Job drawing, mm, ordinate dimensions from the low corner. One solid piece. A direction names the side the tool comes from. Coordinates: 2 decimals unless noted, no trailing zeros. Order: outer loops, then holes, each group sorted by start corner. A loop starts at its lowest first (then second) coordinate and runs counter-clockwise, first axis right, second up. Notation, with made-up numbers: (78, -21) -> (99, -21) arc R26 cw to (99, 2) -> close; hole circle Ø6 at (3.5, 48.5). An arc over 180 degrees is marked (long way). Use CSV: the item, a comma, the result in double quotes. Start each with the question number.
(1) Cut at C-C on y = 13. Write the cut outline in (x, z), plus the area to 3 significant figures.
(2) Cut at D-D on y = 5.5. Write the cut outline in (x, z) (3 decimals), plus the area to 3 significant figures.
(3) Cut at B-B on z = 17.5. Write the cut outline in (x, y) (3 decimals).
(4) Tool access for the marked faces 4 and 5: list every direction of +Z, -Z, +X, -X, +Y, -Y with a clear straight run to the whole face (end or side of a thin tool).
(5) Cut at A-A on x = 17.5. Write the cut outline in (y, z) (3 decimals).
(6) Pin check, flat tips, straight feed: pin 1 Ø8 at (x, z) = (17.5, 17.5) entering from -Y; pin 2 Ø3 at (x, y) = (11.5, 4.5) entering from +Z; pin 3 Ø8 at (x, y) = (24.5, 12) entering from +Z. Stop position of each tip, or through.
(7) Probe L1, parallel to Y at x = 26, z = 13.5; L2, parallel to Z at x = 17.5, y = 5.25 (3 decimals); L3, parallel to Z at x = 17.5, y = 16.5 (3 decimals). List the from-to ranges inside material, lowest first.
(8) Pull direction X, two halves, no side cores. Call the marked faces 1, 2 and 3: pulls with the +X half, pulls with the -X half, needs draft (parallel to the pull), parting line crosses it, or undercut.
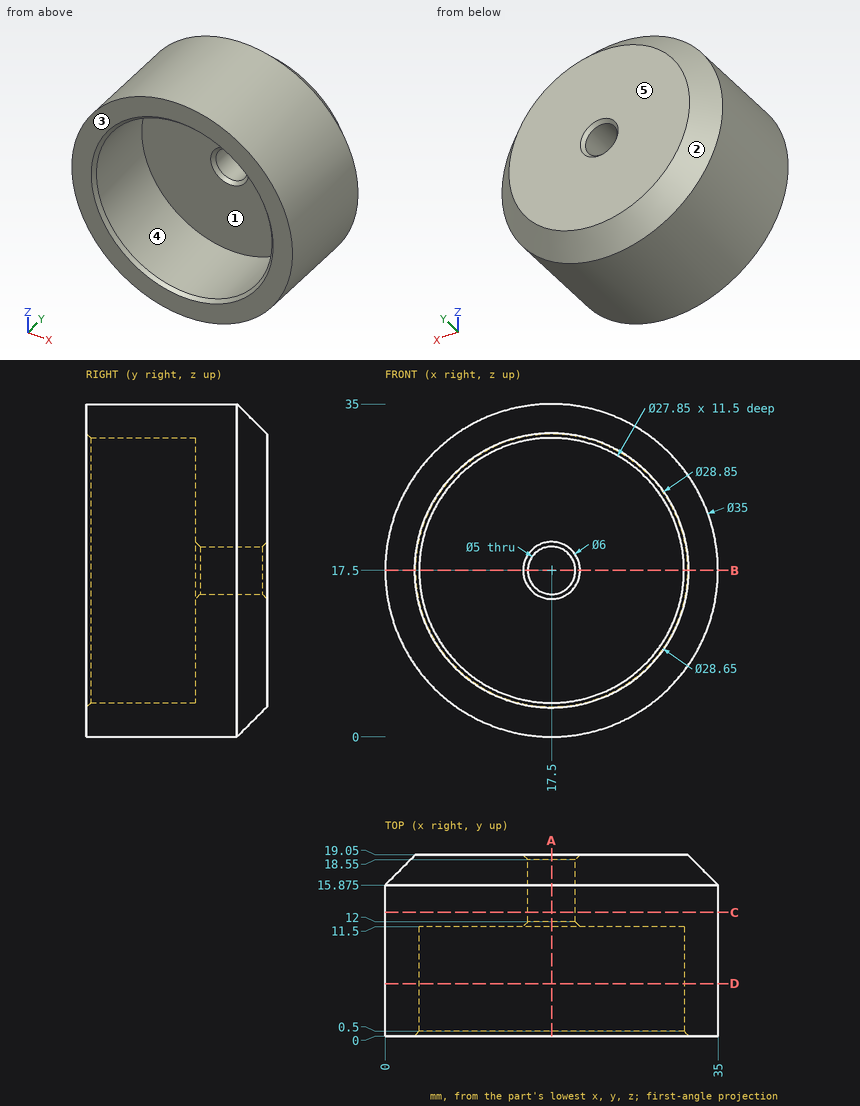
Outcome:
1,outline,"circle Ø35 at (17.5, 17.5); hole circle Ø5 at (17.5, 17.5)"
1,area,"942 mm2"
2,outline,"circle Ø35 at (17.5, 17.5); hole circle Ø27.85 at (17.5, 17.5)"
2,area,"353 mm2"
3,outline,"(0, 0) -> (3.075, 0) -> (3.575, 0.5) -> (3.575, 11.5) -> (14.5, 11.5) -> (15, 12) -> (15, 18.55) -> (14.5, 19.05) -> (3.175, 19.05) -> (0, 15.875) -> close; (20, 12) -> (20.5, 11.5) -> (31.425, 11.5) -> (31.425, 0.5) -> (31.925, 0) -> (35, 0) -> (35, 15.875) -> (31.825, 19.05) -> (20.5, 19.05) -> (20, 18.55) -> close"
4,face 4,"-Y"
4,face 5,"+Z, -Z, +X, -X, +Y"
5,outline,"(0, 0) -> (15.875, 0) -> (19.05, 3.175) -> (19.05, 14.5) -> (18.55, 15) -> (12, 15) -> (11.5, 14.5) -> (11.5, 3.575) -> (0.5, 3.575) -> (0, 3.075) -> close; (0, 31.925) -> (0.5, 31.425) -> (11.5, 31.425) -> (11.5, 20.5) -> (12, 20) -> (18.55, 20) -> (19.05, 20.5) -> (19.05, 31.825) -> (15.875, 35) -> (0, 35) -> close"
6,pin 1,"y = 11.5"
6,pin 2,"z = 34.41"
6,pin 3,"z = 34.74"
7,L1,"11.5 to 19.05"
7,L2,"0 to 3.575, 31.425 to 35"
7,L3,"0.625 to 15, 20 to 34.375"
8,face 1,"undercut"
8,face 2,"parting line crosses it"
8,face 3,"needs draft"
